CAD build for the part. Positions are in the model's coordinates, mm. A direction names the side the tool comes from. Give positions to 0.01 mm unless a question says otherwise; leave off trailing zeros. Write each loop counter-clockwise with the first axis right and the second up, starting at its lowest first coordinate (ties: lowest second). Pieces come first, ordered by that corner, then holes. Notation, with made-up numbers: (25, -39) - (79, -39) arc R23 ccw to (79, -9) - close; hole circle Ø5 at (11.25, 84). An arc over 180 degrees is marked (long way). Answer as a JSON object with one key per item and string values.
from build123d import *

# Parameters (mm, degrees)
SKETCH_1_W               = 43.2
SKETCH_1_H               = 27.5
EXTRUDE_1_DEPTH          = 2
CUT_EXTRUDE_1_REACH      = 27.683
SKETCH_2_R               = 1.65
CUT_EXTRUDE_2_REACH      = 27.683
MIRROR_2_COPY_1_REACH    = 27.683
MIRROR_2_COPY_1_SKETCH_R = 1.65
MIRROR_2_COPY_2_REACH    = 27.683
CUT_EXTRUDE_3_REACH      = 27.683
SKETCH_4_R               = 4


with BuildPart() as part:
    # 草图1 → 凸台-拉伸1 (new body)
    with BuildSketch(Plane(origin=(0, 0, 0), x_dir=(1, 0, 0), z_dir=(0, 1, 0))):
        Rectangle(SKETCH_1_W, SKETCH_1_H)
    extrude(amount=EXTRUDE_1_DEPTH)

    # 草图2 → 切除-拉伸1 (cut, up to next)
    with BuildSketch(Plane(origin=(0, 2, 0), x_dir=(1, 0, 0), z_dir=(0, 1, 0)), mode=Mode.PRIVATE) as cut_extrude_1_sk1:
        with Locations(Location((-17, 9, 0), (0, 0, 270))):
            Circle(SKETCH_2_R)
    cut_extrude_1_tool1 = extrude(cut_extrude_1_sk1.sketch, amount=-CUT_EXTRUDE_1_REACH, mode=Mode.PRIVATE) & part.part
    cut_extrude_1 = cut_extrude_1_tool1.solids().sort_by_distance((-17, 2, -9))[0]
    add(cut_extrude_1, mode=Mode.SUBTRACT)

    # 草图3 → 切除-拉伸2 (cut, up to next)
    with BuildSketch(Plane(origin=(0, 2, 0), x_dir=(1, 0, 0), z_dir=(0, 1, 0)), mode=Mode.PRIVATE) as cut_extrude_2_sk1:
        with BuildLine():
            Line((-6.788225099, 4.5254834), (-10.033845225, 7.771103525))
            ThreePointArc((-10.033845225, 7.771103525), (-10.033845225, 10.033845225), (-7.771103525, 10.033845225))
            Line((-7.771103525, 10.033845225), (-4.5254834, 6.788225099))
            ThreePointArc((-4.5254834, 6.788225099), (-4.5254834, 4.5254834), (-6.788225099, 4.5254834))
        make_face()
    cut_extrude_2_tool1 = extrude(cut_extrude_2_sk1.sketch, amount=-CUT_EXTRUDE_2_REACH, mode=Mode.PRIVATE) & part.part
    cut_extrude_2 = cut_extrude_2_tool1.solids().sort_by_distance((-7.279664, 2, -7.279664))[0]
    add(cut_extrude_2, mode=Mode.SUBTRACT)

    # 镜向1: 切除-拉伸1, 切除-拉伸2 across plane
    add(cut_extrude_1.mirror(Plane.XY), mode=Mode.SUBTRACT)
    add(cut_extrude_2.mirror(Plane.XY), mode=Mode.SUBTRACT)

    # 镜向2: 切除-拉伸1, 切除-拉伸2 across plane
    add(cut_extrude_1.mirror(Plane(origin=(0, 0, 0), x_dir=(0, 0, 1), z_dir=(1, 0, 0))), mode=Mode.SUBTRACT)
    add(cut_extrude_2.mirror(Plane(origin=(0, 0, 0), x_dir=(0, 0, 1), z_dir=(1, 0, 0))), mode=Mode.SUBTRACT)

    # 镜向2 copy 1 sketch → 镜向2 copy 1 (cut, up to next)
    with BuildSketch(Plane(origin=(0, 2, 0), x_dir=(-1, 0, 0), z_dir=(0, 1, 0)), mode=Mode.PRIVATE) as mirror_2_copy_1_sk1:
        with Locations(Location((-17, 9, 0), (0, 0, 270))):
            Circle(MIRROR_2_COPY_1_SKETCH_R)
    mirror_2_copy_1_tool1 = extrude(mirror_2_copy_1_sk1.sketch, amount=-MIRROR_2_COPY_1_REACH, mode=Mode.PRIVATE) & part.part
    add(mirror_2_copy_1_tool1.solids().sort_by_distance((17, 2, 9))[0], mode=Mode.SUBTRACT)

    # 镜向2 copy 2 sketch → 镜向2 copy 2 (cut, up to next)
    with BuildSketch(Plane(origin=(0, 2, 0), x_dir=(-1, 0, 0), z_dir=(0, 1, 0)), mode=Mode.PRIVATE) as mirror_2_copy_2_sk1:
        with BuildLine():
            Line((-6.788225099, 4.5254834), (-10.033845225, 7.771103525))
            ThreePointArc((-10.033845225, 7.771103525), (-10.033845225, 10.033845225), (-7.771103525, 10.033845225))
            Line((-7.771103525, 10.033845225), (-4.5254834, 6.788225099))
            ThreePointArc((-4.5254834, 6.788225099), (-4.5254834, 4.5254834), (-6.788225099, 4.5254834))
        make_face()
    mirror_2_copy_2_tool1 = extrude(mirror_2_copy_2_sk1.sketch, amount=-MIRROR_2_COPY_2_REACH, mode=Mode.PRIVATE) & part.part
    add(mirror_2_copy_2_tool1.solids().sort_by_distance((7.279664, 2, 7.279664))[0], mode=Mode.SUBTRACT)

    # 草图4 → 切除-拉伸3 (cut, up to next)
    with BuildSketch(Plane(origin=(0, 2, 0), x_dir=(1, 0, 0), z_dir=(0, 1, 0)), mode=Mode.PRIVATE) as cut_extrude_3_sk1:
        with Locations(Location((0, 0, 0), (0, 0, 270))):
            Circle(SKETCH_4_R)
    cut_extrude_3_tool1 = extrude(cut_extrude_3_sk1.sketch, amount=-CUT_EXTRUDE_3_REACH, mode=Mode.PRIVATE) & part.part
    add(cut_extrude_3_tool1.solids().sort_by_distance((0, 2, 0))[0], mode=Mode.SUBTRACT)


solid = part.part
Item 1: Cut at D-D (z = 0). Give the cut face in (x, y).
Entries:
{"outline": "(-21.6, 0) - (-4, 0) - (-4, 2) - (-21.6, 2) - close; (4, 0) - (21.6, 0) - (21.6, 2) - (4, 2) - close"}
Item 2: Cut at A-A (x = -17). Give the cut face in (y, z).
Entries:
{"outline": "(0, -13.75) - (2, -13.75) - (2, -10.65) - (0, -10.65) - close; (0, -7.35) - (2, -7.35) - (2, 7.35) - (0, 7.35) - close; (0, 10.65) - (2, 10.65) - (2, 13.75) - (0, 13.75) - close"}
Item 3: Probe line 1 (Z direction, x = 17, y = 0.9); line 2 (X direction, y = 1.4, z = -9); line 3 (X direction, y = 1.5, z = 4.5). List the from-to ranges inside material, lowest first. Write a range as from..to.
Entries:
{"line 1": "-13.75..-10.65, -7.35..7.35, 10.65..13.75", "line 2": "-21.6..-18.65, -15.35..-10.5, -6.74..6.74, 10.5..15.35, 18.65..21.6", "line 3": "-21.6..-6.76, -4.55..4.55, 6.76..21.6"}
Item 4: Which spindle directions (+Z, -Z, +X, -X, +Y, -Y) get a long thin tool onto all of the face, cutting with end or side? Do faces 1 (the flat face through (6.17, 1.01, 8.43)), 2 (the flat face through (0, 1, -13.75)). Say none if no direction does.
Entries:
{"face 1": "+Y, -Y", "face 2": "-Z, +X, -X, +Y, -Y"}
Item 5: Cut at C-C (x = 0). Give the cut face in (y, z), and give its area (3 significant figures).
Entries:
{"outline": "(0, -13.75) - (2, -13.75) - (2, -4) - (0, -4) - close; (0, 4) - (2, 4) - (2, 13.75) - (0, 13.75) - close", "area": "39.0 mm2"}
Item 6: Mould opens along X. For faces 3 (the flat face through (-5, 0, 0)), 4 (the flat face through (-21.6, 1, 0)), 5 (the flat face through (6.17, 1.01, -8.43)) say: +X half, -X half, draft (parallel to the pull), parting line (faces both ways), or undercut.
Entries:
{"face 3": "draft", "face 4": "-X half", "face 5": "undercut"}
Item 7: Cut at B-B (y = 1.2). State how many separate pieces and enclosed holes the cut face has, and give its area (3 significant figures).
Entries:
{"separate pieces": "1", "enclosed holes": "9", "area": "1,010 mm2"}
